Check sheet for the modelled part. Datum: model origin and axes. Units: mm. A direction names the side the tool comes from. Coordinates: 2 decimals unless noted, no trailing zeros. Loops run counter-clockwise (first coordinate to the right, second up) from the corner with the lowest first, then second, coordinate; pieces in that order, holes last. Notation, with made-up numbers: M 35.25,54 L 76.25,54 A9 cw 76.25,67 Z; hole C 36.25,-24.5 d7. An arc over 180 degrees is marked long. Answer in a Markdown table with one row per item. Add a question column.
```python
from build123d import *

# Parameters (mm, degrees)
F0_W     = 100
F0_H     = 20
F1_DEPTH = 15
F3_DEPTH = 20
F4_R     = 5


with BuildPart() as f1:
    # F0 (on Front) → F1 (new body)
    with BuildSketch(Plane.XZ):
        Rectangle(F0_W, F0_H)
    extrude(amount=F1_DEPTH)

    # F2 (on face) → F3 (cut, through all)
    with BuildSketch(Plane.XY.offset(10)):
        with BuildLine():
            Line((-37.5, -15), (-37.673208, -14.301388))
            Line((-37.673208, -14.301388), (-39.001597, -8.943505))
            ThreePointArc((-39.001597, -8.943505), (-40, -8), (-40.998403, -8.943505))
            Line((-40.998403, -8.943505), (-42.5, -15))
            Line((-42.5, -15), (-37.5, -15))
        make_face()
        with BuildLine():
            Line((-29.5, -15), (-29.673208, -14.301388))
            Line((-29.673208, -14.301388), (-31.001597, -8.943505))
            ThreePointArc((-31.001597, -8.943505), (-32, -8), (-32.998403, -8.943505))
            Line((-32.998403, -8.943505), (-34.348484, -14.388879))
            Line((-34.348484, -14.388879), (-34.5, -15))
            Line((-34.5, -15), (-29.5, -15))
        make_face()
        with BuildLine():
            Line((-21.5, -15), (-21.673208, -14.301388))
            Line((-21.673208, -14.301388), (-23.001597, -8.943505))
            ThreePointArc((-23.001597, -8.943505), (-24, -8), (-24.998403, -8.943505))
            Line((-24.998403, -8.943505), (-26.348484, -14.388879))
            Line((-26.348484, -14.388879), (-26.5, -15))
            Line((-26.5, -15), (-21.5, -15))
        make_face()
        with BuildLine():
            Line((-13.5, -15), (-13.673208, -14.301388))
            Line((-13.673208, -14.301388), (-15.001597, -8.943505))
            ThreePointArc((-15.001597, -8.943505), (-16, -8), (-16.998403, -8.943505))
            Line((-16.998403, -8.943505), (-18.348484, -14.388879))
            Line((-18.348484, -14.388879), (-18.5, -15))
            Line((-18.5, -15), (-13.5, -15))
        make_face()
        with BuildLine():
            Line((-5.5, -15), (-5.673208, -14.301388))
            Line((-5.673208, -14.301388), (-7.001597, -8.943505))
            ThreePointArc((-7.001597, -8.943505), (-8, -8), (-8.998403, -8.943505))
            Line((-8.998403, -8.943505), (-10.348484, -14.388879))
            Line((-10.348484, -14.388879), (-10.5, -15))
            Line((-10.5, -15), (-5.5, -15))
        make_face()
        with BuildLine():
            Line((2.326792, -14.301388), (0.998403, -8.943505))
            ThreePointArc((0.998403, -8.943505), (0, -8), (-0.998403, -8.943505))
            Line((-0.998403, -8.943505), (-2.348484, -14.388879))
            Line((-2.348484, -14.388879), (-2.5, -15))
            Line((-2.5, -15), (2.5, -15))
            Line((2.5, -15), (2.326792, -14.301388))
        make_face()
        with BuildLine():
            Line((7.001597, -8.943505), (5.651516, -14.388879))
            Line((5.651516, -14.388879), (5.5, -15))
            Line((5.5, -15), (10.5, -15))
            Line((10.5, -15), (10.326792, -14.301388))
            Line((10.326792, -14.301388), (8.998403, -8.943505))
            ThreePointArc((8.998403, -8.943505), (8, -8), (7.001597, -8.943505))
        make_face()
        with BuildLine():
            Line((15.001597, -8.943505), (13.651516, -14.388879))
            Line((13.651516, -14.388879), (13.5, -15))
            Line((13.5, -15), (18.5, -15))
            Line((18.5, -15), (18.326792, -14.301388))
            Line((18.326792, -14.301388), (16.998403, -8.943505))
            ThreePointArc((16.998403, -8.943505), (16, -8), (15.001597, -8.943505))
        make_face()
        with BuildLine():
            Line((23.001597, -8.943505), (21.651516, -14.388879))
            Line((21.651516, -14.388879), (21.5, -15))
            Line((21.5, -15), (26.5, -15))
            Line((26.5, -15), (26.326792, -14.301388))
            Line((26.326792, -14.301388), (24.998403, -8.943505))
            ThreePointArc((24.998403, -8.943505), (24, -8), (23.001597, -8.943505))
        make_face()
        with BuildLine():
            Line((31.001597, -8.943505), (29.651516, -14.388879))
            Line((29.651516, -14.388879), (29.5, -15))
            Line((29.5, -15), (34.5, -15))
            Line((34.5, -15), (34.326792, -14.301388))
            Line((34.326792, -14.301388), (32.998403, -8.943505))
            ThreePointArc((32.998403, -8.943505), (32, -8), (31.001597, -8.943505))
        make_face()
        with BuildLine():
            Line((39.001597, -8.943505), (37.651516, -14.388879))
            Line((37.651516, -14.388879), (37.5, -15))
            Line((37.5, -15), (42.5, -15))
            Line((42.5, -15), (40.998403, -8.943505))
            ThreePointArc((40.998403, -8.943505), (40, -8), (39.001597, -8.943505))
        make_face()
        with BuildLine():
            ThreePointArc((13.651516, -14.388879), (13.026891, -14.800623), (12.305824, -15))
            Line((12.305824, -15), (13.5, -15))
            Line((13.5, -15), (13.651516, -14.388879))
        make_face()
        with BuildLine():
            Line((10.326792, -14.301388), (10.5, -15))
            Line((10.5, -15), (11.763503, -15))
            ThreePointArc((11.763503, -15), (10.985304, -14.773765), (10.326792, -14.301388))
        make_face()
        with BuildLine():
            Line((18.326792, -14.301388), (18.5, -15))
            Line((18.5, -15), (19.763503, -15))
            ThreePointArc((19.763503, -15), (18.985304, -14.773765), (18.326792, -14.301388))
        make_face()
        with BuildLine():
            ThreePointArc((21.651516, -14.388879), (21.026891, -14.800623), (20.305824, -15))
            Line((20.305824, -15), (21.5, -15))
            Line((21.5, -15), (21.651516, -14.388879))
        make_face()
        with BuildLine():
            Line((26.326792, -14.301388), (26.5, -15))
            Line((26.5, -15), (27.763503, -15))
            ThreePointArc((27.763503, -15), (26.985304, -14.773765), (26.326792, -14.301388))
        make_face()
        with BuildLine():
            ThreePointArc((29.651516, -14.388879), (29.026891, -14.800623), (28.305824, -15))
            Line((28.305824, -15), (29.5, -15))
            Line((29.5, -15), (29.651516, -14.388879))
        make_face()
        with BuildLine():
            Line((34.326792, -14.301388), (34.5, -15))
            Line((34.5, -15), (35.763503, -15))
            ThreePointArc((35.763503, -15), (34.985304, -14.773765), (34.326792, -14.301388))
        make_face()
        with BuildLine():
            ThreePointArc((37.651516, -14.388879), (37.026891, -14.800623), (36.305824, -15))
            Line((36.305824, -15), (37.5, -15))
            Line((37.5, -15), (37.651516, -14.388879))
        make_face()
        with BuildLine():
            ThreePointArc((5.651516, -14.388879), (5.026891, -14.800623), (4.305824, -15))
            Line((4.305824, -15), (5.5, -15))
            Line((5.5, -15), (5.651516, -14.388879))
        make_face()
        with BuildLine():
            ThreePointArc((3.763503, -15), (2.985304, -14.773765), (2.326792, -14.301388))
            Line((2.326792, -14.301388), (2.5, -15))
            Line((2.5, -15), (3.763503, -15))
        make_face()
        with BuildLine():
            Line((-2.5, -15), (-2.348484, -14.388879))
            ThreePointArc((-2.348484, -14.388879), (-2.973109, -14.800623), (-3.694176, -15))
            Line((-3.694176, -15), (-2.5, -15))
        make_face()
        with BuildLine():
            Line((-5.5, -15), (-4.236497, -15))
            ThreePointArc((-4.236497, -15), (-5.014696, -14.773765), (-5.673208, -14.301388))
            Line((-5.673208, -14.301388), (-5.5, -15))
        make_face()
        with BuildLine():
            Line((-11.694176, -15), (-10.5, -15))
            Line((-10.5, -15), (-10.348484, -14.388879))
            ThreePointArc((-10.348484, -14.388879), (-10.973109, -14.800623), (-11.694176, -15))
        make_face()
        with BuildLine():
            Line((-13.5, -15), (-12.236497, -15))
            ThreePointArc((-12.236497, -15), (-13.014696, -14.773765), (-13.673208, -14.301388))
            Line((-13.673208, -14.301388), (-13.5, -15))
        make_face()
        with BuildLine():
            Line((-19.694176, -15), (-18.5, -15))
            Line((-18.5, -15), (-18.348484, -14.388879))
            ThreePointArc((-18.348484, -14.388879), (-18.973109, -14.800623), (-19.694176, -15))
        make_face()
        with BuildLine():
            Line((-21.5, -15), (-20.236497, -15))
            ThreePointArc((-20.236497, -15), (-21.014696, -14.773765), (-21.673208, -14.301388))
            Line((-21.673208, -14.301388), (-21.5, -15))
        make_face()
        with BuildLine():
            Line((-27.694176, -15), (-26.5, -15))
            Line((-26.5, -15), (-26.348484, -14.388879))
            ThreePointArc((-26.348484, -14.388879), (-26.973109, -14.800623), (-27.694176, -15))
        make_face()
        with BuildLine():
            Line((-29.5, -15), (-28.236497, -15))
            ThreePointArc((-28.236497, -15), (-29.014696, -14.773765), (-29.673208, -14.301388))
            Line((-29.673208, -14.301388), (-29.5, -15))
        make_face()
        with BuildLine():
            Line((-35.694176, -15), (-34.5, -15))
            Line((-34.5, -15), (-34.348484, -14.388879))
            ThreePointArc((-34.348484, -14.388879), (-34.973109, -14.800623), (-35.694176, -15))
        make_face()
        with BuildLine():
            Line((-37.5, -15), (-36.236497, -15))
            ThreePointArc((-36.236497, -15), (-37.014696, -14.773765), (-37.673208, -14.301388))
            Line((-37.673208, -14.301388), (-37.5, -15))
        make_face()
    extrude(amount=-F3_DEPTH, mode=Mode.SUBTRACT)

    # F4
    f4_edges = [f1.edges().sort_by_distance(p)[0] for p in [
        (-50, -15, 0),
        (50, -15, 0),
    ]]
    fillet(f4_edges, radius=F4_R)


solid = f1.part
```
Q1. Cross-section at A-A (x = 32). Record the cut outline in (y, z), plus the area to 3 significant figures.
Q2. Cross-section at B-B (y = -11). Count the separate pieces of the cut face and the enclosed holes in it, plus the area to 3 significant figures.
Q3. Go/stop test with a flat-tipped pin: pin 1 (10 mm diameter, centred on x = -11, z = -7, fed in from -Y). Record where the tip stops, or that it passes through.
Q4. Thickness scan on L1, parallel to Y at x = -8, z = -8; L2, parallel to Y at x = 35, z = -6. Record the ranges inside material, lowest first.
Q5. Mould release check, pull along X, two halves, no side actions. Record for faces 3 (the face through (49, -13, 0)), 4 (the face through (-38.33, -11.66, 0.14)), 5 (the face through (-1, 0, 0)): released by +X, released by -X, zero draft, split by the parting line, or undercut.
Q6. Access from +Z, -Z, +X, -X, +Y, -Y to the whole of each face (thin tool, end or side, straight path). Record for faces 1 (the face through (-30.33, -11.66, 0.14)), 2 (the face through (-44, -15, 0)).
Answer key:
| question | item | result |
|---|---|---|
| 1 | outline | M -8,-10 L 0,-10 L 0,10 L -8,10 Z |
| 1 | area | 160 mm^2 |
| 2 | separate pieces | 12 |
| 2 | enclosed holes | 0 |
| 2 | area | 1,330 mm^2 |
| 3 | pin 1 | y = -15 |
| 4 | L1 | -8 to 0 |
| 4 | L2 | -14.78 to 0 |
| 5 | face 3 | released by +X |
| 5 | face 4 | undercut |
| 5 | face 5 | zero draft |
| 6 | face 1 | +Z, -Z, -Y |
| 6 | face 2 | +Z, -Z, +X, -X, -Y |
